Print and shaded views of the part. All mm, measured from the part's lowest x, y and z. Coordinates: 2 decimals unless noted, no trailing zeros. Order: outer loops, then holes, each group sorted by start corner. A loop starts at its lowest first (then second) coordinate and runs counter-clockwise, first axis right, second up.
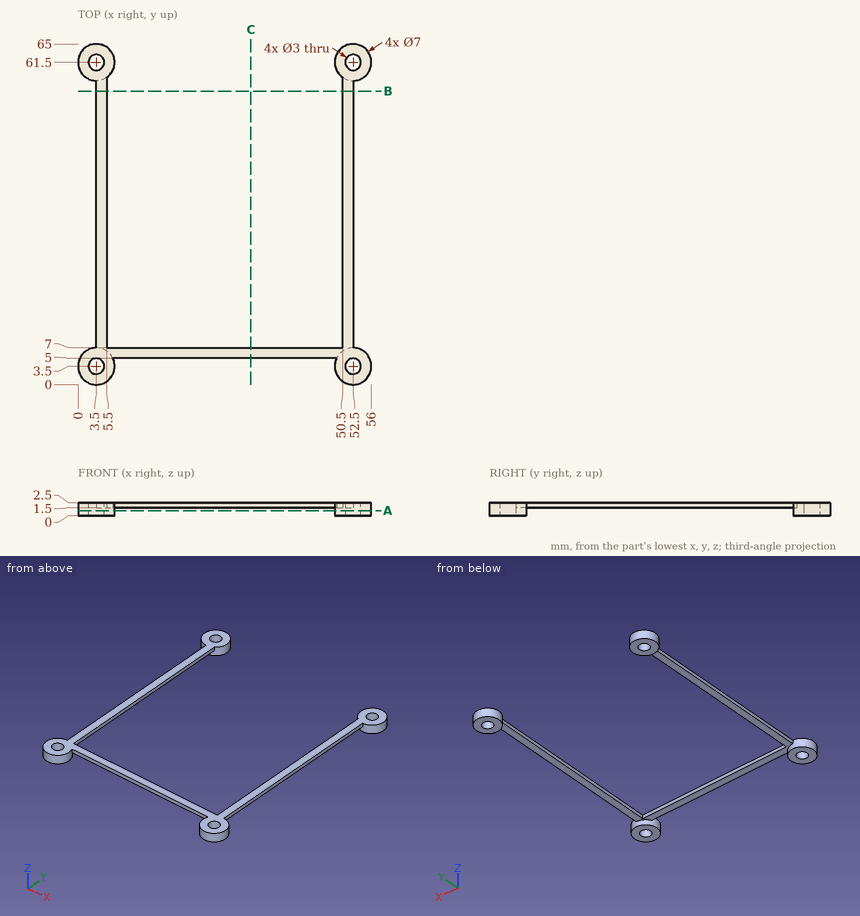
Q1. Cut at B-B, the plane y = 56. List the corners of the cut face in (x, z), plus the area to 3 significant figures.
Established:
outline: (3.5, 1.5) - (5.5, 1.5) - (5.5, 2.5) - (3.5, 2.5) - close; (50.5, 1.5) - (52.5, 1.5) - (52.5, 2.5) - (50.5, 2.5) - close
area: 4.00 mm2
Q2. Probe line 1 (Y direction, x = 52.5, z = 1.3); line 2 (X direction, y = 61.5, z = 0.5); line 3 (X direction, y = 23.5, z = 1.7). List the from-to ranges inside material, lowest first.
Established:
line 1: y = 0 to 2, 5 to 7, 58 to 60, 63 to 65
line 2: x = 0 to 2, 5 to 7, 49 to 51, 54 to 56
line 3: x = 3.5 to 5.5, 50.5 to 52.5
Q3. Drop flat-ended pins along their axis: P1, Ø0.8, axis at y = 35, z = 2, coming from the +X side; P2, Ø1.5, axis at y = 28.5, z = 1, coming from the -X side; P3, Ø2.5, axis at x = 52.5, y = 3.5, coming from the +Z side; P4, Ø0.5, axis at x = 35, z = 2, coming from the +Y side. Give the stop position or say it passes through.
Established:
P1: stops at x = 52.5
P2: stops at x = 3.5
P3: passes through
P4: stops at y = 7
Q4. Cut at A-A, the plane z = 0.95. List the corners of the cut face in (x, y), plus the area to 3 significant figures.
Established:
outline: circle Ø7 at (3.5, 3.5); circle Ø7 at (3.5, 61.5); circle Ø7 at (52.5, 3.5); circle Ø7 at (52.5, 61.5); hole circle Ø3 at (3.5, 3.5); hole circle Ø3 at (3.5, 61.5); hole circle Ø3 at (52.5, 3.5); hole circle Ø3 at (52.5, 61.5)
area: 126 mm2
Q5. Cut at C-C, the plane x = 33. List the corners of the cut face in (y, z).
Established:
outline: (5, 1.5) - (7, 1.5) - (7, 2.5) - (5, 2.5) - close
